from build123d import *

# Parameters (mm, degrees)
BOSS_EXTRUDE1_DEPTH        = 25
F_1_2_0_5_DIAMETER_HOLE1_D = 12.7


with BuildPart() as part:
    # Sketch1 → Boss-Extrude1 (new, symmetric)
    with BuildSketch(Plane(origin=(0, 0, 0), x_dir=(0, 0, -1), z_dir=(1, 0, 0))):
        with BuildLine():
            Line((0, -30), (0, -60))
            Line((0, -60), (20, -60))
            Line((20, -60), (20, -31.721443851))
            ThreePointArc((20, -31.721443851), (37.5, 0), (20, 31.721443851))
            Line((20, 31.721443851), (20, 60))
            Line((20, 60), (0, 60))
            Line((0, 60), (0, 30))
            ThreePointArc((0, 30), (30, 0), (0, -30))
        make_face()
    extrude(amount=BOSS_EXTRUDE1_DEPTH, both=True)

    # 1/2 (0.5) Diameter Hole1 (through all)
    with Locations(Plane.XY):
        with Locations((-15, 45), (15, 45), (15, -45), (-15, -45)):
            Hole(F_1_2_0_5_DIAMETER_HOLE1_D / 2)


solid = part.part
The listing builds one solid part. Answer for the finished solid, in the listing's coordinates (mm). A direction names the side the tool comes from. Round coordinates to 2 decimals unless told otherwise and drop trailing zeros. Write each loop counter-clockwise with the first axis right and the second up, starting at its lowest first coordinate (ties: lowest second). Pieces come first, ordered by that corner, then holes. Notation, with made-up numbers: M 58.5,56 L 102.5,56 A14 ccw 102.5,72 Z; hole C 31,57 d7. An arc over 180 degrees is marked long. Write each question's results on one line, items separated by ' | '. Start each with the question number.
Item 1: For a pull along Y with two mould halves and no side action, classify faces 4 (the face through (-25, 1, -31)), 5 (the face through (-17.93, 39.366, -10.14)), 6 (the face through (0, 60, -10)) as pulls with the +Y half, pulls with the -Y half, needs draft (parallel to the pull), parting line crosses it, or undercut.
Item 2: For faces 1 (the face through (16.38, 38.8, -10.14)), 2 (the face through (0, -46, -20)), 3 (the face through (0, 46, -20)), determine the directions among +Z, -Z, +X, -X, +Y, -Y from which every point of the face is accessible in a straight line to the end or side of a thin tool.
Item 3: A cutting plane is placed at C-C on x = 6. Write down the section's boundary in (y, z).
Item 4: Straight lines are drawn through the part: L1, parallel to Y at x = 15, z = -12; L2, parallel to Y at x = -15, z = -15; L3, parallel to X at y = -41.5, z = -8. For each, find the intervals that lie inside material, in ascending order. Write a range as [from, to].
Item 5: A cutting plane is placed at A-A on z = -9. Write down the section's boundary in (x, y), and give its area (3 significant figures).
Item 6: A cutting plane is placed at D-D on x = 20. Write down the section's boundary in (y, z).
Item 7: A cutting plane is placed at B-B on y = -45. Write down the section's boundary in (x, z), and give its area (3 significant figures).
Item 8: Flat-ended cylindrical pins translate along their axes: pin 1 Ø16.5 at (x, y) = (15, 45) entering from -Z; pin 2 Ø12 at (x, z) = (7.5, -28.5) entering from -Y; pin 3 Ø10 at (x, y) = (-17.5, -6) entering from +Z; pin 4 Ø10 at (x, y) = (-15, -45) entering from +Z. Find the tip coordinate at first contact, or state that the pin passes through.
Check sheet entries:
1) face 4: needs draft | face 5: undercut | face 6: pulls with the +Y half
2) face 1: +Z, -Z | face 2: -Z, +X, -X, -Y | face 3: -Z, +X, -X, +Y
3) outline: M -60,-20 L -31.72,-20 A37.5 ccw 31.72,-20 L 60,-20 L 60,0 L 30,0 A30 cw -30,0 L -60,0 Z
4) L1: [-60, -51.35], [-38.65, -27.5], [27.5, 38.65], [51.35, 60] | L2: [-60, -51.35], [-38.65, -25.98], [25.98, 38.65], [51.35, 60] | L3: [-25, -20.3], [-9.7, 9.7], [20.3, 25]
5) outline: M -25,-60 L 25,-60 L 25,-28.62 L -25,-28.62 Z; M -25,28.62 L 25,28.62 L 25,60 L -25,60 Z; hole C -15,-45 d12.7; hole C -15,45 d12.7; hole C 15,-45 d12.7; hole C 15,45 d12.7 | area: 2,630 mm²
6) outline: M -60,-20 L -48.91,-20 L -48.91,0 L -60,0 Z; M -41.09,-20 L -31.72,-20 A37.5 ccw 31.72,-20 L 41.09,-20 L 41.09,0 L 30,0 A30 cw -30,0 L -41.09,0 Z; M 48.91,-20 L 60,-20 L 60,0 L 48.91,0 Z
7) outline: M -25,-20 L -21.35,-20 L -21.35,0 L -25,0 Z; M -8.65,-20 L 8.65,-20 L 8.65,0 L -8.65,0 Z; M 21.35,-20 L 25,-20 L 25,0 L 21.35,0 Z | area: 492 mm²
8) pin 1: z = -20 | pin 2: y = -30 | pin 3: z = -27.91 | pin 4: through
